Part model, mm, in its own coordinate system. Coordinates: 2 decimals unless noted, no trailing zeros. Order: outer loops, then holes, each group sorted by start corner. A loop starts at its lowest first (then second) coordinate and runs counter-clockwise, first axis right, second up.
1) Cut at A-A (y = -5.5). List the corners of the cut face in (x, z).
2) Cut at D-D (z = 96.5). List the corners of the cut face in (x, y).
3) Wall check: L1, parallel to Z at x = 332.5, y = -5.5; L2, parallel to X at y = -14.25, z = 25.5; L3, parallel to Y at x = 229.5, z = 60 (3 decimals). Give the ranges that are in metal, low to high.
4) Cut at C-C (z = 58). List the corners of the cut face in (x, y) (3 decimals).
5) Pin check, flat tips, straight feed: pin 1 Ø5.5 at (y, z) = (-14, 83) entering from -X; pin 2 Ø7.5 at (y, z) = (-3, 63) entering from +X; pin 3 Ø15 at (x, z) = (247, 59) entering from +Y (3 decimals). Stop position of each tip, or through.
6) Cut at B-B (x = 187). List the corners of the cut face in (y, z) (3 decimals), and give its area (3 significant figures).
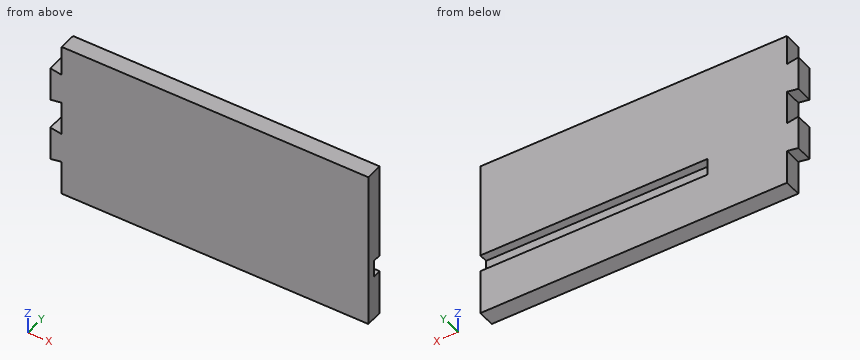
```python
from build123d import *

# Parameters (mm, degrees)
F1_DEPTH = 19.05
F2_W     = 254
F2_H     = 19.05
F3_DEPTH = 9.525


with BuildPart() as f1:
    # F0 (on Front) → F1 (new body)
    with BuildSketch(Plane.XZ):
        Polygon((12.7, 38.468058), (12.7, 0), (355.6, 0), (355.6, 177.8), (12.7, 177.8), (12.7, 143.810647), (0, 146.05), (0, 107.95), (12.7, 110.189353), (12.7, 72.089353), (0, 74.328705), (0, 36.228705), align=None)
    extrude(amount=F1_DEPTH)

    # F2 (on face) → F3 (cut)
    with BuildSketch(Plane(origin=(0, 0, 0), x_dir=(-1, 0, 0), z_dir=(0, 1, 0))):
        with Locations((-228.6, 60.325)):
            Rectangle(F2_W, F2_H)
    extrude(amount=-F3_DEPTH, mode=Mode.SUBTRACT)


solid = f1.part
```
Geometry check:
1. outline: (0, 36.23) - (12.7, 38.47) - (12.7, 0) - (355.6, 0) - (355.6, 50.8) - (101.6, 50.8) - (101.6, 69.85) - (355.6, 69.85) - (355.6, 177.8) - (12.7, 177.8) - (12.7, 143.81) - (0, 146.05) - (0, 107.95) - (12.7, 110.19) - (12.7, 72.09) - (0, 74.33) - close
2. outline: (12.7, -19.05) - (355.6, -19.05) - (355.6, 0) - (12.7, 0) - close
3. L1: z = 0 to 50.8, 69.85 to 177.8
3. L2: x = 12.7 to 355.6
3. L3: y = -19.05 to -9.525
4. outline: (0, -19.05) - (355.6, -19.05) - (355.6, -9.525) - (101.6, -9.525) - (101.6, 0) - (0, 0) - close
5. pin 1: stops at x = 12.7
5. pin 2: stops at x = 101.6
5. pin 3: stops at y = -9.525
6. outline: (-19.05, 0) - (0, 0) - (0, 50.8) - (-9.525, 50.8) - (-9.525, 69.85) - (0, 69.85) - (0, 177.8) - (-19.05, 177.8) - close
6. area: 3,210 mm2
